```python
from build123d import *

# Parameters (mm, degrees)
F0_R     = 3.5
F0_R_2   = 15.25
F1_DEPTH = 2
F2_R     = 28.6
F3_DEPTH = 2
F4_R     = 5
F5_DEPTH = 1


with BuildPart() as f1:
    # F0 (on Front) → F1 (new body)
    with BuildSketch(Plane.XZ):
        with BuildLine():
            Line((-21.58884, 40.619232), (-42.861558, 29.312929))
            ThreePointArc((-42.861558, 29.312929), (-44.997448, 27.729855), (-46.388978, 25.46451))
            Line((-46.388978, 25.46451), (-53.672966, 6.783229))
            Line((-53.672966, 6.783229), (-53.864057, 6.293138))
            ThreePointArc((-53.864057, 6.293138), (-53.705851, -6.701832), (-44.839242, -16.20328))
            ThreePointArc((-44.839242, -16.20328), (-43.103725, -17.591673), (-42.141379, -19.595055))
            Line((-42.141379, -19.595055), (-38.205048, -36.897988))
            ThreePointArc((-38.205048, -36.897988), (-35.569679, -41.232337), (-30.857548, -43.110523))
            Line((-30.857548, -43.110523), (-30.043042, -43.115206))
            Line((-30.043042, -43.115206), (-9.797797, -43.231604))
            ThreePointArc((-9.797797, -43.231604), (-7.190907, -43.98259), (-5.359933, -45.984437))
            ThreePointArc((-5.359933, -45.984437), (-0.034496, -49.287837), (5.328573, -46.04589))
            ThreePointArc((5.328573, -46.04589), (7.182444, -44.065228), (9.797797, -43.344267))
            Line((9.797797, -43.344267), (28.65177, -43.452666))
            ThreePointArc((28.65177, -43.452666), (33.085897, -42.033009), (35.827873, -38.270234))
            Line((35.827873, -38.270234), (41.995789, -19.285684))
            ThreePointArc((41.995789, -19.285684), (43.003835, -17.520371), (44.631304, -16.302245))
            ThreePointArc((44.631304, -16.302245), (54.75181, -2.9788), (49.534597, 12.918354))
            ThreePointArc((49.534597, 12.918354), (48.411586, 14.558602), (48.01643, 16.506786))
            Line((48.01643, 16.506786), (48.01643, 22.9754))
            ThreePointArc((48.01643, 22.9754), (47.987621, 23.511359), (47.901529, 24.041142))
            ThreePointArc((47.901529, 24.041142), (44.750848, 28.885488), (39.182116, 30.429409))
            ThreePointArc((39.182116, 30.429409), (38.635854, 30.360699), (38.095468, 30.255318))
            ThreePointArc((38.095468, 30.255318), (37.863026, 30.207571), (37.628581, 30.170906))
            ThreePointArc((37.628581, 30.170906), (35.306998, 30.413689), (33.348619, 31.683901))
            ThreePointArc((33.348619, 31.683901), (7.384655, 45.403379), (-21.58884, 40.619232))
        make_face()
        with Locations((-30.40436, -35.12337)):
            Circle(F0_R, mode=Mode.SUBTRACT)
        with Locations((28.69489, -35.95279)):
            Circle(F0_R, mode=Mode.SUBTRACT)
        with Locations((-39.83717, 23)):
            Circle(F0_R, mode=Mode.SUBTRACT)
        Circle(F0_R_2, mode=Mode.SUBTRACT)
        with Locations((39.55455, 23.39376)):
            Circle(F0_R, mode=Mode.SUBTRACT)
        with BuildLine():
            Line((-53.864057, 6.293138), (-53.672966, 6.783229))
            ThreePointArc((-53.672966, 6.783229), (-53.770302, 6.538881), (-53.864057, 6.293138))
        make_face()
        with BuildLine():
            ThreePointArc((39.182116, 30.429409), (38.398103, 30.343702), (37.628581, 30.170906))
            ThreePointArc((37.628581, 30.170906), (37.863026, 30.207571), (38.095468, 30.255318))
            ThreePointArc((38.095468, 30.255318), (38.635854, 30.360699), (39.182116, 30.429409))
        make_face()
        with BuildLine():
            Line((-30.043042, -43.115206), (-30.857548, -43.110523))
            ThreePointArc((-30.857548, -43.110523), (-30.450354, -43.123238), (-30.043042, -43.115206))
        make_face()
    extrude(amount=F1_DEPTH)

    # F2 (on face) → F3 (join)
    with BuildSketch(Plane(origin=(0, 0, 0), x_dir=(-1, 0, 0), z_dir=(0, 1, 0))):
        with BuildLine():
            ThreePointArc((-37.097917, 9.914867), (-48.4, 0), (-37.097917, -9.914867))
            ThreePointArc((-37.097917, -9.914867), (38.4, 0), (-37.097917, 9.914867))
        make_face()
        Circle(F2_R, mode=Mode.SUBTRACT)
    extrude(amount=F3_DEPTH)

    # F4 (on face) → F5 (cut)
    with BuildSketch(Plane.XZ.offset(2)):
        with Locations((-39.83717, 23)):
            Circle(F4_R)
        with Locations((39.55455, 23.39376)):
            Circle(F4_R)
        with Locations((28.69489, -35.95279)):
            Circle(F4_R)
        with Locations((-30.40436, -35.12337)):
            Circle(F4_R)
    extrude(amount=-F5_DEPTH, mode=Mode.SUBTRACT)


solid = f1.part
```
Work out the finished part from the listing and answer in its coordinate system (mm). A direction names the side the tool comes from. Give positions to 0.01 mm unless a question says otherwise; leave off trailing zeros. Order: outer loops, then holes, each group sorted by start corner. A loop starts at its lowest first (then second) coordinate and runs counter-clockwise, first axis right, second up.
1. Section A-A, the plane x = 0 is taken. Determine the outline of the cut face in (y, z), and give its area (3 significant figures).
Result sheet:
outline: (-2, -49.29) - (0, -49.29) - (0, -38.4) - (2, -38.4) - (2, -28.6) - (0, -28.6) - (0, -15.25) - (-2, -15.25) - close; (-2, 15.25) - (0, 15.25) - (0, 28.6) - (2, 28.6) - (2, 38.4) - (0, 38.4) - (0, 46) - (-2, 46) - close
area: 169 mm2
2. Section C-C, the plane x = -18 is taken. Determine the outline of the cut face in (y, z).
Result sheet:
outline: (-2, -43.18) - (0, -43.18) - (0, -33.92) - (2, -33.92) - (2, -22.23) - (0, -22.23) - (0, 22.23) - (2, 22.23) - (2, 33.92) - (0, 33.92) - (0, 42.33) - (-2, 42.33) - close
3. Straight lines are drawn through the part: L1, parallel to Y at x = 20.5, z = -13; L2, parallel to Z at x = 0, y = -1.35; L3, parallel to Z at x = -5.5, y = -0.2. For each, find the intervals that lie inside material, in ascending order.
Result sheet:
L1: y = -2 to 0
L2: z = -49.29 to -15.25, 15.25 to 46
L3: z = -45.73 to -14.22, 14.22 to 45.67
4. Section B-B, the plane z = 0 is taken. Determine the outline of the cut face in (x, y).
Result sheet:
outline: (-55, -2) - (-15.25, -2) - (-15.25, 0) - (-28.6, 0) - (-28.6, 2) - (-38.4, 2) - (-38.4, 0) - (-55, 0) - close; (15.25, -2) - (55, -2) - (55, 0) - (48.4, 0) - (48.4, 2) - (28.6, 2) - (28.6, 0) - (15.25, 0) - close
5. Section D-D, the plane y = 0.8 is taken. Determine the outline of the cut face in (x, z), and give its area (3 significant figures).
Result sheet:
outline: (37.1, -9.91) arc R10 ccw (long way) to (37.1, 9.91) arc R38.4 ccw (long way) to start; hole circle Ø57.2 at (0, 0)
area: 2,230 mm2
6. Each of these flat-tipped pins is pushed along its axis until it touches: P1, Ø13, axis at x = 28.69, z = -35.95, coming from the +Y side; P2, Ø6, axis at x = 39.55, z = 23.39, coming from the -Y side; P3, Ø1, axis at x = 20.5, y = 1, coming from the -Z side; P4, Ø9, axis at x = -30.4, z = -35.12, coming from the -Y side. Where does it stop, or does it pass through?
Result sheet:
P1: stops at y = 0
P2: passes through
P3: stops at z = -32.78
P4: stops at y = -1
7. The mould has two halves that part along X. Classify faces 1 (the flat face through (28, 2, -8)), 2 (the cylindrical face through (-35.62, -0.99, -41.19)), 3 (the flat face through (25, -1, -37)): released by +X, released by -X, zero draft, split by the parting line, or undercut.
Result sheet:
face 1: zero draft
face 2: released by -X
face 3: undercut
8. For faces 4 (the flat face through (-37.7, -1, 19.7)), 5 (the cylindrical face through (42.89, -0.49, 24.45)), 6 (the cylindrical face through (7.15, -0.986, -44.085)), determine the directions among +Z, -Z, +X, -X, +Y, -Y from which every point of the face is accessible in a straight line to the end or side of a thin tool.
Result sheet:
face 4: -Y
face 5: +Y, -Y
face 6: -Z, +Y, -Y
